Geometry check sheet. Reference: drawing and pictorial views, mm from the part's lowest x, y, z. A direction names the side the tool comes from. Give positions to 0.01 mm unless a question says otherwise; leave off trailing zeros. Loops run counter-clockwise (first coordinate to the right, second up) from the corner with the lowest first, then second, coordinate; pieces in that order, holes last. Notation, with made-up numbers: (1.25, 9) - (47.25, 9) arc R4 cw to (47.25, 13) - close; hole circle Ø6 at (42.5, 51.25). An arc over 180 degrees is marked (long way). One line per question, with ' | ' between items. Start each with the question number.
1. Section check C-C, the plane z = 3.5. Enter the section's corners in (x, y).
2. Thickness scan on line 1 along Z through (x, y) = (10, 2.5); line 2 along Y through (x, z) = (18, 3.5); line 3 along X through (y, z) = (21.5, 5.25). Record the ranges inside material, lowest first. Write a range as from..to.
3. Section check A-A, the plane x = 18. Enter the section's corners in (y, z).
4. Depth check by flat-ended pin: pin 1 Ø1 at (x, z) = (11.5, 4) entering from -Y; pin 2 Ø1.5 at (x, z) = (25.5, 5) entering from +Y; pin 3 Ø1 at (x, z) = (28, 4.5) entering from -Y. Enter the tip coordinate at first touch or a pass-through.
5. Mould release check, pull along Z, two halves, no side actions. Record for the marked faces 3, 4 and 5: +Z half, -Z half, draft (parallel to the pull), parting line (faces both ways), or undercut.
6. Section check D-D, the plane z = 0.5. Enter the section's corners in (x, y).
7. Tool access check on the marked faces 1 and 2. Record the directions out of +Z, -Z, +X, -X, +Y, -Y that give a thin tool (end or side, any length) a straight path to the whole face; none if there is none.
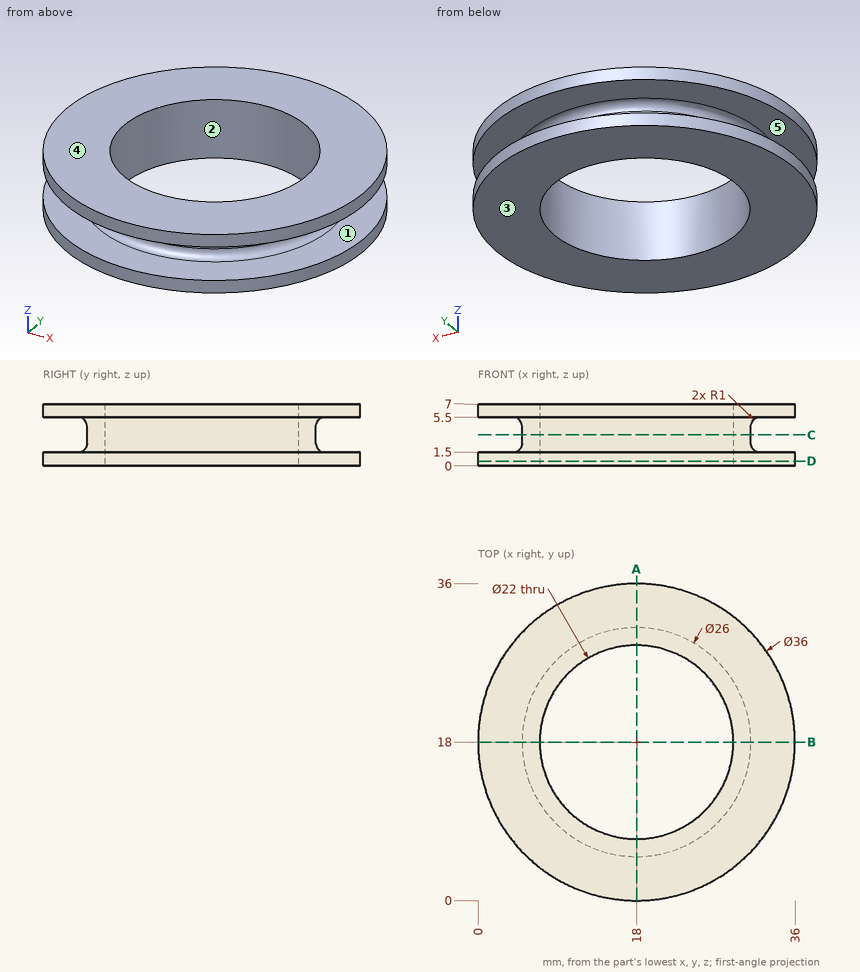
Results list:
1) outline: circle Ø26 at (18, 18); hole circle Ø22 at (18, 18)
2) line 1: 0..1.5, 5.5..7 | line 2: 5..7, 29..31 | line 3: 5.13..7.57, 28.43..30.87
3) outline: (0, 0) - (7, 0) - (7, 7) - (0, 7) - (0, 5.5) - (4, 5.5) arc R1 cw to (5, 4.5) - (5, 2.5) arc R1 cw to (4, 1.5) - (0, 1.5) - close; (29, 0) - (36, 0) - (36, 1.5) - (32, 1.5) arc R1 cw to (31, 2.5) - (31, 4.5) arc R1 cw to (32, 5.5) - (36, 5.5) - (36, 7) - (29, 7) - close
4) pin 1: y = 6.47 | pin 2: y = 34.61 | pin 3: y = 9.13
5) face 3: -Z half | face 4: +Z half | face 5: undercut
6) outline: circle Ø36 at (18, 18); hole circle Ø22 at (18, 18)
7) face 1: none | face 2: +Z, -Z
